Source: CAD feature listing. Evaluate the final solid. Frame: model axes, mm. A direction names the side the tool comes from. Give positions to 0.01 mm unless a question says otherwise; leave off trailing zeros. Order: outer loops, then holes, each group sorted by start corner. A loop starts at its lowest first (then second) coordinate and runs counter-clockwise, first axis right, second up. Notation, with made-up numbers: M 30.25,42.25 L 70.25,42.25 A30 ccw 70.25,66.25 Z; hole C 44,38.5 d6. An arc over 180 degrees is marked long. Return JSON: item names as keys, results as strings.
Autodesk Inventor part; units mm, degrees
ref_plane "Плоскость сечения" through (-4.509, 19.8692, 0) normal (-0.9752, -0.2213, 0) x (0, 0, 1)
ref_plane "РабПлоскость2" through (0, 0, 0) normal (-1, 0, 0) x (0, 0, 1)
ref_plane "РабПлоскость3" through (-55.5305, 0, 0) normal (0.9298, -0.3681, 0) x (0, 0, 1)
sketch "Эскизная траектория" plane through (0, 0, 0) normal (0, 0, 1) x (1, 0, 0)
  arc A0 (-4.509, -19.8692) -> (-4.509, 19.8692) centre (0, 0) ccw
  arc A1 (-57.3198, 7.8846) -> (-57.3198, -7.8846) centre (-55.5305, 0) ccw
  line L0 (-57.3198, 7.8846) -> (-4.509, 19.8692)
  line L1 (-4.509, -19.8692) -> (-57.3198, -7.8846)
ref_plane "Плоскость сечения" through (-4.509, 19.8692, 0) normal (-0.9752, -0.2213, 0) x (0, 0, 1)
ref_plane "РабПлоскость2" through (0, 0, 0) normal (-1, 0, 0) x (0, 0, 1)
ref_plane "РабПлоскость3" through (-55.5305, 0, 0) normal (0.9298, -0.3681, 0) x (0, 0, 1)
sketch "Сечение" plane through (-4.509, 19.8692, 0) normal (-0.9752, -0.2213, 0) x (0, 0, 1)
  line L0 (-3.175, 0.381) -> (3.175, 0.381)
  line L1 (3.175, 0.381) -> (3.175, -0.254)
  line L2 (3.175, -0.254) -> (-3.175, -0.254)
  line L3 (-3.175, -0.254) -> (-3.175, 0.381)
  line L4 (-3.175, 0) -> (3.175, 0) construction
  point P0 (0, 0)
  point P1 (0, 0)
  dimension "d0" = 6.35
  dimension "d4" = 0.254
  dimension "d5" = 0.381
sweep "Ремень" add profiles "Сечение" path "Эскизная траектория"
equation "\"d0\" = da_B"
equation "\"d4\" = da_a"
equation "\"d5\" = da_a2"
equation "\"da_B\" = 6.35"
equation "\"da_pb\" = 2.032"
equation "\"da_L\" = 203.2"
equation "\"da_a\" = 0.254"
equation "\"da_S\" = 1.143"
equation "\"da_Beta\" = 20deg"
equation "\"da_Ht\" = 0.508"
equation "\"da_H\" = 1.143"
equation "\"da_a2\" = 0.381"
properties part number "Зубчатый ремень" material "Rubber"
1. Draft query along X for faces 3 (the face through (-31.368, 14.165, 0.044)), 4 (the face through (-30.489, -13.713, -0.044)), 5 (the face through (-7.42, 19.13, 3.175)), 6 (the face through (-31.228, 13.545, -0.044)). Return one class per face: pulls with the +X half, pulls with the -X half, needs draft (parallel to the pull), parting line crosses it, or undercut.
Evaluation:
{"face 3": "pulls with the -X half", "face 4": "undercut", "face 5": "needs draft", "face 6": "undercut"}
2. Section query B-B (y = 0). Return loops of the section in (x, z) (3 decimals).
Evaluation:
{"outline": "M -63.997,-3.175 L -63.362,-3.175 L -63.362,3.175 L -63.997,3.175 Z; M 20.12,-3.175 L 20.755,-3.175 L 20.755,3.175 L 20.12,3.175 Z"}
3. Set-up query: faces 1 (the face through (-63.36, 0.15, 0.04)), 2 (the face through (-30.629, -14.332, 0.044)). Return all of +Z, -Z, +X, -X, +Y, -Y with unobstructed straight access to the full face (end or side cutting, diameter ignored); none if empty.
Evaluation:
{"face 1": "+Z, -Z", "face 2": "+Z, -Z, -X, -Y"}
4. Section query C-C (z = 1). Return loops of the section in (x, y), then the cut area to 3 significant figures.
Evaluation:
{"outline": "M -57.4,-8.26 L -4.59,-20.24 A20.76 ccw long -4.59,20.24 L -57.4,8.26 A8.47 ccw Z; hole M -57.26,-7.64 L -4.45,-19.62 A20.12 ccw long -4.45,19.62 L -57.26,7.64 A7.83 ccw Z", "area": "129 mm^2"}
5. Ray query, probe 1 along Y at (x, z) = (0, 1); probe 2 along X at (y, z) = (-6.5, 1.75); probe 3 along Y at (x, z) = (-15, -2.75). Return the intervals inside material, ascending.
Evaluation:
{"probe 1": "y = -20.76 to -20.12, 20.12 to 20.76", "probe 2": "x = -60.95 to -59.9, 19.04 to 19.71", "probe 3": "y = -17.88 to -17.23, 17.23 to 17.88"}
6. First-contact query: pin 1 (3 mm diameter, centred on y = -5, z = 2.5, fed in from -X); pin 2 (1.5 mm diameter, centred on x = -25, z = 2.5, fed in from +Y); pin 3 (1 mm diameter, centred on x = -24, z = 2, fed in from +Y). Flat tips, straight axial feed; report the tip coordinate or a pass-through.
Evaluation:
{"pin 1": "stops at x = -63.24", "pin 2": "stops at y = 15.78", "pin 3": "stops at y = 15.95"}
7. Section query A-A (x = 0). Return loops of the section in (y, z) (3 decimals).
Evaluation:
{"outline": "M -20.755,-3.175 L -20.12,-3.175 L -20.12,3.175 L -20.755,3.175 Z; M 20.12,-3.175 L 20.755,-3.175 L 20.755,3.175 L 20.12,3.175 Z"}
